Design review of the part built by this model. Coordinates are the model's own, in mm. Face numbers are marked on the shaded views. Give positions to 0.01 mm unless a question says otherwise; leave off trailing zeros. Write each loop counter-clockwise with the first axis right and the second up, starting at its lowest first coordinate (ties: lowest second). Pieces come first, ordered by that corner, then holes. Notation, with made-up numbers: M 22,81.5 L 48,81.5 A13 ccw 48,105.5 Z; hole C 38,-14 d9. An arc over 180 degrees is marked long. Use a Markdown table: item, result. Add a question column.
```python
from build123d import *


with BuildPart() as f1:
    # F0 (on Front) → F1 (revolve)
    with BuildSketch(Plane.XZ):
        with BuildLine():
            Line((-4.991404, 27.199442), (-4.991404, 0))
            Line((-4.991404, 0), (35.008596, 0))
            Line((35.008596, 0), (52.980236, 24.937051))
            ThreePointArc((52.980236, 24.937051), (54.598683, 28.136221), (55.156134, 31.677874))
            Line((55.156134, 31.677874), (55.156134, 36.973636))
            ThreePointArc((55.156134, 36.973636), (54.70711, 39.319052), (53.423542, 41.332769))
            Line((53.423542, 41.332769), (48.533764, 59.208133))
            Line((48.533764, 59.208133), (60.298596, 86.575069))
            Line((60.298596, 86.575069), (60.298596, 93.405227))
            Line((60.298596, 93.405227), (47.884241, 93.482569))
            Line((47.884241, 93.482569), (35.008596, 71.05868))
            Line((35.008596, 71.05868), (0, 27.199442))
            Line((0, 27.199442), (-4.991404, 27.199442))
        make_face()
    revolve(axis=Axis((-4.991404, 0, 50.455429), (0, 0, 1)))


solid = f1.part
```
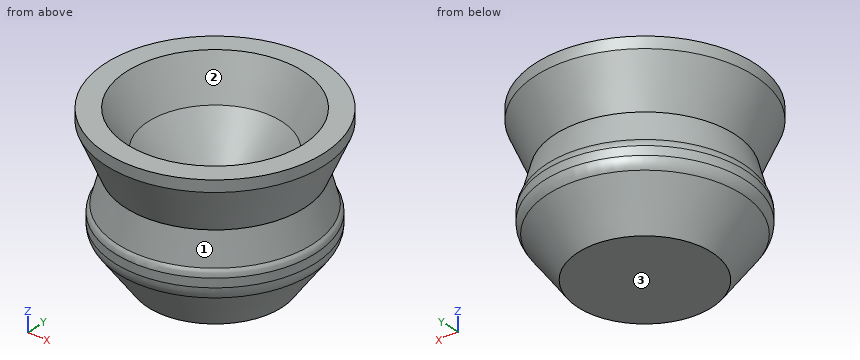
(1) Add section A-A on y = 0. Give the boundary of the cut face in (x, z).
(2) For pin 1 (8 mm diameter, centred on x = 27, y = -50.5, fed in from +Z); pin 2 (10 mm diameter, centred on y = 5, z = 57, fed in from -X); pin 3 (1.5 mm diameter, centred on x = 44.5, z = 44.5, fed in from -Y), all flat-tipped, find the tip position at first contact; note any pin that passes through.
(3) Add section B-B on z = 75.5. Give the boundary of the cut face in (x, y).
(4) The part is to be moulded in two halves that separate along Y. For the marked faces 1, 2 and 3, say which applies: released by +Y, released by -Y, zero draft, split by the parting line, or undercut.
(5) Add section C-C on z = 7.5. Give the boundary of the cut face in (x, y), then the cut area to 3 significant figures.
(6) Wall thickness on L1, parallel to Y at x = 1, z = 66.5; L2, parallel to Y at x = 9, z = 43; L3, parallel to Z at x = -34.5, y = 19.5: over which ranges is each line inside the solid? List them lowest first.
From the geometry:
| question | item | result |
|---|---|---|
| 1 | outline | M -70.28,86.58 L -58.52,59.21 L -63.41,41.33 A6.35 ccw -65.14,36.97 L -65.14,31.68 A11.53 ccw -62.96,24.94 L -44.99,0 L 35.01,0 L 52.98,24.94 A11.53 ccw 55.16,31.68 L 55.16,36.97 A6.35 ccw 53.42,41.33 L 48.53,59.21 L 60.3,86.58 L 60.3,93.41 L 47.88,93.48 L 35.01,71.06 L 0,27.2 L -9.98,27.2 L -44.99,71.06 L -57.87,93.48 L -70.28,93.41 Z |
| 2 | pin 1 | stops at z = 93.46 |
| 2 | pin 2 | stops at x = -60.32 |
| 2 | pin 3 | stops at y = -30.66 |
| 3 | outline | C -4.99,0 d121.06; hole C -4.99,0 d85.1 |
| 4 | face 1 | split by the parting line |
| 4 | face 2 | undercut |
| 4 | face 3 | zero draft |
| 5 | outline | C -4.99,0 d90.81 |
| 5 | area | 6,480 mm^2 |
| 6 | L1 | y = -56.34 to -35.86, 35.86 to 56.34 |
| 6 | L2 | y = -56.24 to -10.68, 10.68 to 56.24 |
| 6 | L3 | z = 0 to 65.26 |
